For this review, take the finished solid that the model builds, in its own axes (mm). A direction names the side the tool comes from. Round coordinates to 2 decimals unless told otherwise and drop trailing zeros. Loops run counter-clockwise (first coordinate to the right, second up) from the corner with the lowest first, then second, coordinate; pieces in that order, holes last. Notation, with made-up numbers: (8, -5.5) -> (52, -5.5) arc R16 ccw to (52, 7.5) -> close; hole circle Ø10 at (21, 77). An arc over 180 degrees is marked (long way). Use one line per item in the form item = value. Start each with the question number.
from build123d import *

# Parameters (mm, degrees)
SKETCH1_W               = 11.8
SKETCH1_H               = 18
BOSS_EXTRUDE1_DEPTH     = 1.19
SKETCH2_W               = 10.5
SKETCH2_H               = 13.46
BOSS_EXTRUDE2_DEPTH     = 3.2
FILLET11_R              = 0.5
FILLET12_R              = 0.5
FILLET13_R              = 0.5
FILLET14_R              = 0.5
SKETCH9_R               = 0.3
CUT_EXTRUDE5_DEPTH      = 3.2
SKETCH14_W              = 5.1
SKETCH14_H              = 2
BOSS_EXTRUDE3_DEPTH     = 3.2
SKETCH15_W              = 3.9
SKETCH15_H              = 2
BOSS_EXTRUDE4_DEPTH     = 3.3
SKETCH16_R              = 0.3
CUT_EXTRUDE6_DEPTH      = 4.3
CUT_EXTRUDE6_DEPTH_BACK = 1
SKETCH17_R              = 0.3
CUT_EXTRUDE9_DEPTH      = 4.3
CUT_EXTRUDE9_DEPTH_BACK = 3.2
SKETCH19_W              = 1.11
SKETCH19_H              = 0.5
BOSS_EXTRUDE6_DEPTH     = 1.6
SKETCH20_W              = 1.11
SKETCH20_H              = 0.5
BOSS_EXTRUDE7_DEPTH     = 1.6


with BuildPart() as part:
    # Sketch1 → Boss-Extrude1 (new body)
    with BuildSketch(Plane.XY):
        with Locations((5.9, 9)):
            Rectangle(SKETCH1_W, SKETCH1_H)
    extrude(amount=BOSS_EXTRUDE1_DEPTH)

    # Sketch2 → Boss-Extrude2 (add)
    with BuildSketch(Plane.XY):
        with Locations((5.9, 7.23)):
            Rectangle(SKETCH2_W, SKETCH2_H)
    extrude(amount=BOSS_EXTRUDE2_DEPTH)

    # Fillet11
    fillet11_edges = [part.edges().sort_by_distance(p)[0] for p in [
        (0.65, 13.96, 2.195),
    ]]
    fillet(fillet11_edges, radius=FILLET11_R)

    # Fillet12
    fillet12_edges = [part.edges().sort_by_distance(p)[0] for p in [
        (0.65, 0.5, 2.195),
    ]]
    fillet(fillet12_edges, radius=FILLET12_R)

    # Fillet13
    fillet13_edges = [part.edges().sort_by_distance(p)[0] for p in [
        (11.15, 0.5, 2.195),
    ]]
    fillet(fillet13_edges, radius=FILLET13_R)

    # Fillet14
    fillet14_edges = [part.edges().sort_by_distance(p)[0] for p in [
        (11.15, 13.96, 2.195),
    ]]
    fillet(fillet14_edges, radius=FILLET14_R)

    # Sketch9 → Cut-Extrude5 (cut)
    with BuildSketch(Plane.XY):
        with Locations((1.1, -0.15)):
            Circle(SKETCH9_R)
        with Locations((1.9, -0.15)):
            Circle(SKETCH9_R)
        with Locations((2.7, -0.15)):
            Circle(SKETCH9_R)
        with Locations((3.5, -0.15)):
            Circle(SKETCH9_R)
        with Locations((4.3, -0.15)):
            Circle(SKETCH9_R)
        with Locations((5.1, -0.15)):
            Circle(SKETCH9_R)
        with Locations((5.9, -0.15)):
            Circle(SKETCH9_R)
        with Locations((6.7, -0.15)):
            Circle(SKETCH9_R)
        with Locations((7.5, -0.15)):
            Circle(SKETCH9_R)
        with Locations((8.3, -0.15)):
            Circle(SKETCH9_R)
        with Locations((9.1, -0.15)):
            Circle(SKETCH9_R)
        with Locations((9.9, -0.15)):
            Circle(SKETCH9_R)
        with Locations((10.7, -0.15)):
            Circle(SKETCH9_R)
    extrude(amount=CUT_EXTRUDE5_DEPTH, mode=Mode.SUBTRACT)

    # Sketch14 → Boss-Extrude3 (add)
    with BuildSketch(Plane.XY):
        with Locations((8.45, 16.312688451)):
            Rectangle(SKETCH14_W, SKETCH14_H)
    extrude(amount=BOSS_EXTRUDE3_DEPTH)

    # Sketch15 → Boss-Extrude4 (add)
    with BuildSketch(Plane.XY):
        with Locations((8.401012654, 16.312688451)):
            Rectangle(SKETCH15_W, SKETCH15_H)
    extrude(amount=BOSS_EXTRUDE4_DEPTH)

    # Sketch16 → Cut-Extrude6 (cut, two sides)
    with BuildSketch(Plane.XY) as cut_extrude6_sk:
        with Locations((-0.15, 1)):
            Circle(SKETCH16_R)
        with Locations((-0.15, 1.8)):
            Circle(SKETCH16_R)
        with Locations((-0.15, 2.6)):
            Circle(SKETCH16_R)
        with Locations((-0.15, 3.4)):
            Circle(SKETCH16_R)
        with Locations((-0.15, 4.2)):
            Circle(SKETCH16_R)
        with Locations((-0.15, 5)):
            Circle(SKETCH16_R)
        with Locations((-0.15, 5.8)):
            Circle(SKETCH16_R)
        with Locations((-0.15, 6.6)):
            Circle(SKETCH16_R)
        with Locations((-0.15, 7.4)):
            Circle(SKETCH16_R)
        with Locations((-0.15, 8.2)):
            Circle(SKETCH16_R)
        with Locations((-0.15, 9)):
            Circle(SKETCH16_R)
        with Locations((-0.15, 9.8)):
            Circle(SKETCH16_R)
        with Locations((-0.15, 10.6)):
            Circle(SKETCH16_R)
        with Locations((-0.15, 11.4)):
            Circle(SKETCH16_R)
        with Locations((-0.15, 12.2)):
            Circle(SKETCH16_R)
        with Locations((-0.15, 13)):
            Circle(SKETCH16_R)
        with Locations((-0.15, 13.8)):
            Circle(SKETCH16_R)
        with Locations((-0.15, 14.6)):
            Circle(SKETCH16_R)
        with Locations((-0.15, 15.4)):
            Circle(SKETCH16_R)
        with Locations((-0.15, 16.2)):
            Circle(SKETCH16_R)
        with Locations((-0.15, 17)):
            Circle(SKETCH16_R)
    extrude(amount=CUT_EXTRUDE6_DEPTH, mode=Mode.SUBTRACT)
    extrude(cut_extrude6_sk.sketch, amount=-CUT_EXTRUDE6_DEPTH_BACK, mode=Mode.SUBTRACT)

    # Sketch17 → Cut-Extrude9 (cut, two sides)
    with BuildSketch(Plane.XY) as cut_extrude9_sk:
        with Locations((11.95, 1)):
            Circle(SKETCH17_R)
        with Locations((11.95, 1.8)):
            Circle(SKETCH17_R)
        with Locations((11.95, 2.6)):
            Circle(SKETCH17_R)
        with Locations((11.95, 3.4)):
            Circle(SKETCH17_R)
        with Locations((11.95, 4.2)):
            Circle(SKETCH17_R)
        with Locations((11.95, 5)):
            Circle(SKETCH17_R)
        with Locations((11.95, 5.8)):
            Circle(SKETCH17_R)
        with Locations((11.95, 6.6)):
            Circle(SKETCH17_R)
        with Locations((11.95, 7.4)):
            Circle(SKETCH17_R)
        with Locations((11.95, 8.2)):
            Circle(SKETCH17_R)
        with Locations((11.95, 9)):
            Circle(SKETCH17_R)
        with Locations((11.95, 9.8)):
            Circle(SKETCH17_R)
        with Locations((11.95, 10.6)):
            Circle(SKETCH17_R)
        with Locations((11.95, 11.4)):
            Circle(SKETCH17_R)
        with Locations((11.95, 12.2)):
            Circle(SKETCH17_R)
        with Locations((11.95, 13)):
            Circle(SKETCH17_R)
        with Locations((11.95, 13.8)):
            Circle(SKETCH17_R)
    extrude(amount=CUT_EXTRUDE9_DEPTH, mode=Mode.SUBTRACT)
    extrude(cut_extrude9_sk.sketch, amount=-CUT_EXTRUDE9_DEPTH_BACK, mode=Mode.SUBTRACT)

    # Sketch19 → Boss-Extrude6 (add)
    with BuildSketch(Plane.XY):
        with Locations((2.875, 16.16471376)):
            Rectangle(SKETCH19_W, SKETCH19_H)
    extrude(amount=BOSS_EXTRUDE6_DEPTH)

    # Sketch20 → Boss-Extrude7 (add)
    with BuildSketch(Plane.XY):
        with Locations((1.55773637, 15.39942892)):
            Rectangle(SKETCH20_W, SKETCH20_H)
    extrude(amount=BOSS_EXTRUDE7_DEPTH)


solid = part.part
Item 1: For P1, Ø1, axis at y = 9, z = 2, coming from the -X side; P2, Ø1, axis at y = 17, z = 2.5, coming from the -X side; P3, Ø0.6, axis at x = 8, z = 2.5, coming from the +Y side, all flat-tipped, find the tip position at first contact; note any pin that passes through.
Item 2: Machinability: for faces 1 (the flat face through (0.65, 7, 2)), 2 (the flat face through (11, 16, 2)), 3 (the flat face through (6, 7, 3.2)), 4 (the flat face through (11.15, 7, 2)), 5 (the flat face through (6, 13.96, 2)), which of the approach directions +Z, -Z, +X, -X, +Y, -Y give a long, thin tool a straight path to every point of the face, cutting with its end or side? Answer none if there is none.
Item 3: Take a section at A-A on z = 2.5. Give the boundary of the cut face in (x, y).
Item 4: Wall thickness on line 1 (Y direction, x = 7.5, z = 1.9); line 2 (Y direction, x = 3.25, z = 2.8); line 3 (Z direction, x = 1.75, y = 2.5): over which ranges is each line inside the solid? List them lowest first.
Item 5: Draft analysis for pull direction Y (two halves, no side actions). For faces 6 (the flat face through (8, 17.313, 2)), 7 (the flat face through (8, 16, 3.3)), 8 (the flat face through (8, 15.313, 2)), state which applies: +Y half, -Y half, draft (parallel to the pull), parting line (faces both ways), or undercut.
Item 6: Take a section at B-B on x = 7.5. Give the boundary of the cut face in (y, z).
Item 7: Take a section at C-C on y = 9.75. Give the boundary of the cut face in (x, z).
Results:
q1.P1 = 0.65
q1.P2 = 5.9
q1.P3 = 17.31
q2.face_1 = +Z, -X, +Y, -Y
q2.face_2 = +Z, +X, +Y
q2.face_3 = +Z, +X, -X, -Y
q2.face_4 = +Z, +X, +Y, -Y
q2.face_5 = +Z, +X, -X
q3.outline = (0.65, 1) arc R0.5 ccw to (1.15, 0.5) -> (10.65, 0.5) arc R0.5 ccw to (11.15, 1) -> (11.15, 13.46) arc R0.5 ccw to (10.65, 13.96) -> (1.15, 13.96) arc R0.5 ccw to (0.65, 13.46) -> close; (5.9, 15.31) -> (11, 15.31) -> (11, 17.31) -> (5.9, 17.31) -> close
q4.line_1 = 0.5 to 13.96, 15.31 to 17.31
q4.line_2 = 0.5 to 13.96
q4.line_3 = 0 to 3.2
q5.face_6 = +Y half
q5.face_7 = draft
q5.face_8 = undercut
q6.outline = (0.15, 0) -> (18, 0) -> (18, 1.19) -> (17.31, 1.19) -> (17.31, 3.3) -> (15.31, 3.3) -> (15.31, 1.19) -> (13.96, 1.19) -> (13.96, 3.2) -> (0.5, 3.2) -> (0.5, 1.19) -> (0.15, 1.19) -> close
q7.outline = (0.15, 0) -> (11.65, 0) -> (11.65, 1.19) -> (11.15, 1.19) -> (11.15, 3.2) -> (0.65, 3.2) -> (0.65, 1.19) -> (0.15, 1.19) -> close
